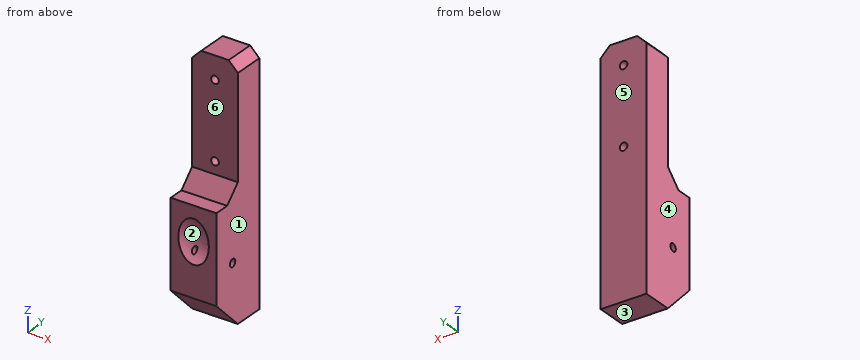
from build123d import *

# Parameters (mm, degrees)
Y_KSEKLIK_EKSTR_ZYON2_DEPTH = 30
IZIM3_R                     = 2.5
KES_EKSTR_ZYON1_DEPTH       = 30
PAH1_SIZE                   = 6
KES_EKSTR_ZYON2_DEPTH       = 30
KES_EKSTR_ZYON2_DEPTH_BACK  = 30
IZIM5_R                     = 10
IZIM6_R                     = 10
KES_EKSTR_ZYON3_DEPTH       = 15
IZIM7_R                     = 2.5
KES_EKSTR_ZYON4_DEPTH       = 48


with BuildPart() as part:
    # izim2 → Y_kseklik-Ekstr_zyon2 (new body)
    with BuildSketch(Plane(origin=(0, 0, 0), x_dir=(0, 0, -1), z_dir=(1, 0, 0))):
        Polygon((-80, 20), (80, 20), (80, 0), (60, -20), (3, -20), (3, -10), (-7, 0), (-80, 0), align=None)
    extrude(amount=Y_KSEKLIK_EKSTR_ZYON2_DEPTH)

    # izim3 → Kes-Ekstr_zyon1 (cut)
    with BuildSketch(Plane(origin=(0, 20, 0), x_dir=(1, 0, 0), z_dir=(0, 1, 0))):
        with Locations(Location((15, -15, 0), (0, 0, 270))):
            Circle(IZIM3_R)
        with Locations(Location((15, -65, 0), (0, 0, 270))):
            Circle(IZIM3_R)
    extrude(amount=-KES_EKSTR_ZYON1_DEPTH, mode=Mode.SUBTRACT)

    # Pah1
    pah1_edges = [part.edges().sort_by_distance(p)[0] for p in [
        (0, 10, 80),
        (30, 10, 80),
    ]]
    chamfer(pah1_edges, length=PAH1_SIZE)

    # izim5 → Kes-Ekstr_zyon2 (cut, two sides: drawn at the far end of the back side and taken through both)
    with BuildSketch(Plane(origin=(0, -3.5, 3.5), x_dir=(1, 0, 0), z_dir=(0, -0.7071067811865488, 0.7071067811865462)).offset(-KES_EKSTR_ZYON2_DEPTH_BACK)):
        with Locations(Location((15, -32, 0), (0, 0, 270))):
            Circle(IZIM5_R)
    extrude(amount=KES_EKSTR_ZYON2_DEPTH + KES_EKSTR_ZYON2_DEPTH_BACK, mode=Mode.SUBTRACT)

    # izim6 → Kes-Ekstr_zyon3 (cut)
    with BuildSketch(Plane(origin=(0, 17.713203436, -17.713203436), x_dir=(1, 0, 0), z_dir=(0, -0.7071067811865488, 0.7071067811865462))):
        with Locations(Location((15, -32, 0), (0, 0, 270))):
            Circle(IZIM6_R)
    extrude(amount=-KES_EKSTR_ZYON3_DEPTH, mode=Mode.SUBTRACT)

    # izim7 → Kes-Ekstr_zyon4 (cut)
    with BuildSketch(Plane(origin=(30, 0, 0), x_dir=(0, 0, -1), z_dir=(1, 0, 0))):
        with Locations((40.340620434, -4.914213562)):
            Circle(IZIM7_R)
    extrude(amount=-KES_EKSTR_ZYON4_DEPTH, mode=Mode.SUBTRACT)


solid = part.part
Design review of the part built by this model. Coordinates are the model's own, in mm. Face numbers are marked on the shaded views. A direction names the side the tool comes from. Coordinates: 2 decimals unless noted, no trailing zeros. Loops run counter-clockwise (first coordinate to the right, second up) from the corner with the lowest first, then second, coordinate; pieces in that order, holes last. Notation, with made-up numbers: (-17, -21) -> (29, -21) arc R30 cw to (29, 4) -> close; hole circle Ø9 at (31.25, 70). An arc over 180 degrees is marked (long way). Use a Markdown table: item, result. Add a question column.
Item 1: We need section C-C, the plane x = 26.5. Write out the cut boundary in (y, z).
Item 2: We need section A-A, the plane x = 15. Write out the cut boundary in (y, z), and give its area (3 significant figures).
Item 3: Wall thickness on L1, parallel to X at y = 9.25, z = 15; L2, parallel to Y at x = 16, z = 61.5; L3, parallel to Z at x = 22, y = 9: over which ranges is each line inside the solid? List them lowest first. Write a range as from..to.
Item 4: We need section D-D, the plane z = 4. Write out the cut boundary in (x, y).
Item 5: Machinability: for the marked faces 5 and 6, which of the approach directions +Z, -Z, +X, -X, +Y, -Y give a long, thin tool a straight path to every point of the face, cutting with its end or side? Answer none if there is none.
Item 6: We need section B-B, the plane z = 65. Write out the cut boundary in (x, y).
Item 7: The part is to be moulded in two halves that separate along X. For the marked faces 1, 2, 3 and 4, say which applies: +X half, -X half, draft (parallel to the pull), parting line (faces both ways), or undercut.
Item 8: Clearance check with flat-ended pins moving along their axes: P1, Ø2, axis at x = 5, z = 10.5, coming from the -Y side; P2, Ø4, axis at y = -4.91, z = -40.34, coming from the -X side; P3, Ø8, axis at x = 11.5, y = -14, coming from the -Z side; P4, Ø6.5, axis at y = -4.91, z = -40.34, coming from the +X side. State where each tip first meets the part, or that it passes through.
Numbers:
| question | item | result |
|---|---|---|
| 1 | outline | (-20, -60) -> (0, -80) -> (20, -80) -> (20, 77.5) -> (0, 77.5) -> (0, 7) -> (-10, -3) -> (-20, -3) -> close; hole circle Ø5 at (-4.91, -40.34) |
| 2 | outline | (-20, -60) -> (0, -80) -> (20, -80) -> (20, 12.5) -> (0, 12.5) -> (0, 7) -> (-10, -3) -> (-20, -3) -> (-20, -11.11) -> (12.76, -43.88) -> (-1.38, -58.02) -> (-20, -39.4) -> close; (0, 17.5) -> (20, 17.5) -> (20, 62.5) -> (0, 62.5) -> close; (0, 67.5) -> (20, 67.5) -> (20, 80) -> (0, 80) -> close |
| 2 | area | 3,660 mm^2 |
| 3 | L1 | x = 0..12.5, 17.5..30 |
| 3 | L2 | y = 0..20 |
| 3 | L3 | z = -80..-47.64, -44.16..80 |
| 4 | outline | (0, -3) -> (30, -3) -> (30, 20) -> (0, 20) -> close |
| 5 | face 5 | +Z, -Z, +X, -X, +Y |
| 5 | face 6 | +Z, +X, -X, -Y |
| 6 | outline | (0, 0) -> (12.5, 0) -> (12.5, 20) -> (0, 20) -> close; (17.5, 0) -> (30, 0) -> (30, 20) -> (17.5, 20) -> close |
| 7 | face 1 | +X half |
| 7 | face 2 | undercut |
| 7 | face 3 | draft |
| 7 | face 4 | -X half |
| 8 | P1 | stops at y = 0 |
| 8 | P2 | passes through |
| 8 | P3 | stops at z = -70 |
| 8 | P4 | stops at x = 30 |
